```python
from build123d import *

# Parameters (mm, degrees)
ESQUISSE1_R             = 30
BOSS_EXTRU_1_DEPTH      = 15
ESQUISSE2_W             = 9.340839883
ESQUISSE2_H             = 53.061818545
ENL_V_MAT_EXTRU_1_DEPTH = 7
ESQUISSE3_W             = 49.4498788
ESQUISSE3_H             = 120
BOSS_EXTRU_2_DEPTH      = 18
ESQUISSE4_R             = 7
ENL_V_MAT_EXTRU_2_DEPTH = 2
ENL_V_MAT_EXTRU_3_DEPTH = 129.01952976
ESQUISSE6_R             = 10
BOSS_EXTRU_3_DEPTH      = 10
ESQUISSE7_W             = 5
ESQUISSE7_H             = 120
ENL_V_MAT_EXTRU_4_DEPTH = 4
D_POUILLE1_ANGLE        = 40


with BuildPart() as part:
    # Esquisse1 → Boss.-Extru.1 (new body)
    with BuildSketch(Plane.XY):
        Circle(ESQUISSE1_R)
    extrude(amount=BOSS_EXTRU_1_DEPTH)

    # Esquisse2 → Enlèv. mat.-Extru.1 (cut)
    with BuildSketch(Plane.XY.offset(15)):
        with Locations((26.230396322, -0.346809271)):
            Rectangle(ESQUISSE2_W, ESQUISSE2_H)
        with Locations((-26.230396322, -0.346809271)):
            Rectangle(ESQUISSE2_W, ESQUISSE2_H)
    extrude(amount=-ENL_V_MAT_EXTRU_1_DEPTH, mode=Mode.SUBTRACT)

    # Esquisse3 → Boss.-Extru.2 (add)
    with BuildSketch(Plane.XY.offset(15)):
        Rectangle(ESQUISSE3_W, ESQUISSE3_H)
    extrude(amount=BOSS_EXTRU_2_DEPTH)

    # Esquisse4 → Enlèv. mat.-Extru.2 (cut)
    with BuildSketch(Plane.XZ.offset(60)):
        with Locations(Location((12.7249394, 24, 0), (0, 0, 270))):
            Circle(ESQUISSE4_R)
        with Locations(Location((-12.7249394, 24, 0), (0, 0, 270))):
            Circle(ESQUISSE4_R)
    enl_v_mat_extru_2 = extrude(amount=-ENL_V_MAT_EXTRU_2_DEPTH, mode=Mode.SUBTRACT)

    # Symétrie1: Enlèv. mat.-Extru.2 across plane
    add(enl_v_mat_extru_2.mirror(Plane.ZX), mode=Mode.SUBTRACT)

    # Esquisse5 → Enlèv. mat.-Extru.3 (cut, through all)
    with BuildSketch(Plane.XZ.offset(60)):
        with BuildLine():
            Line((24.7249394, 18.33578408), (21.356248325, 18.33578408))
            Line((21.356248325, 18.33578408), (21.356248325, 16.410354936))
            Line((21.356248325, 16.410354936), (21.889577151, 16.410354936))
            ThreePointArc((21.889577151, 16.410354936), (22.243130541, 16.263908326), (22.389577151, 15.910354936))
            Line((22.389577151, 15.910354936), (22.389577151, 15))
            Line((22.389577151, 15), (22.700668624, 13.139727122))
            Line((22.700668624, 13.139727122), (26.027148326, 13.139727122))
            Line((26.027148326, 13.139727122), (26.027148326, 18.33578408))
            Line((26.027148326, 18.33578408), (24.7249394, 18.33578408))
        make_face()
        with BuildLine():
            Line((-22.389577151, 15.910354936), (-22.389577151, 15))
            Line((-22.389577151, 15), (-22.389577151, 13.757493185))
            Line((-22.389577151, 13.757493185), (-25.545793937, 13.757493185))
            Line((-25.545793937, 13.757493185), (-25.842888818, 18.33578408))
            Line((-25.842888818, 18.33578408), (-24.7249394, 18.33578408))
            Line((-24.7249394, 18.33578408), (-21.356248325, 18.33578408))
            Line((-21.356248325, 18.33578408), (-21.356248325, 16.410354936))
            Line((-21.356248325, 16.410354936), (-21.889577151, 16.410354936))
            ThreePointArc((-21.889577151, 16.410354936), (-22.243130541, 16.263908326), (-22.389577151, 15.910354936))
        make_face()
    extrude(amount=-ENL_V_MAT_EXTRU_3_DEPTH, mode=Mode.SUBTRACT)

    # Esquisse6 → Boss.-Extru.3 (add)
    with BuildSketch(Plane(origin=(0, 0, 0), x_dir=(-1, 0, 0), z_dir=(0, 0, -1))):
        with Locations(Location((0, 0, 0), (0, 0, 180))):
            Circle(ESQUISSE6_R)
    extrude(amount=BOSS_EXTRU_3_DEPTH)

    # Esquisse7 → Enlèv. mat.-Extru.4 (cut)
    with BuildSketch(Plane.XY.offset(33)):
        Rectangle(ESQUISSE7_W, ESQUISSE7_H)
    extrude(amount=-ENL_V_MAT_EXTRU_4_DEPTH, mode=Mode.SUBTRACT)

    # Dépouille1
    d_pouille1_faces = [part.faces().sort_by_distance(p)[0] for p in [
        (-2.5, 0, 31),
        (2.5, 0, 31),
    ]]
    draft(d_pouille1_faces, Plane(origin=(-2.5, 60, 29), x_dir=(1, 0, 0), z_dir=(0, 0, 1)), D_POUILLE1_ANGLE)


solid = part.part
```
Model file for the job. Use its own axes, mm. A direction names the side the tool comes from. Coordinates: 2 decimals unless noted, no trailing zeros. Loops run counter-clockwise (first coordinate to the right, second up) from the corner with the lowest first, then second, coordinate; pieces in that order, holes last. Notation, with made-up numbers: (82, 25.5) - (117, 25.5) arc R28 ccw to (117, 62.5) - close; hole circle Ø4 at (71.5, 77). An arc over 180 degrees is marked (long way). Write item = value, one per line. Start each with the question number.
Item 1: Drop flat-ended pins along their axis: pin 1 Ø4 at (x, z) = (13, 11.5) entering from +Y; pin 2 Ø6 at (x, y) = (-16.5, -47) entering from -Z; pin 3 Ø1.5 at (x, y) = (-1, 7) entering from +Z. Give the stop position or say it passes through.
Item 2: Saw through at C-C, the plane y = -46.5. List the corners of the cut face in (x, z), then the cut area to 3 significant figures.
Item 3: Saw through at D-D, the plane y = -18. List the corners of the cut face in (x, z).
Item 4: Pull direction Z, two halves, no side cores. Call faces 1 (the face through (13, -58, 24)), 2 (the face through (-4.202, -0.84, 31.028)), 3 (the face through (0, 0, -10)): +Z half, -Z half, draft (parallel to the pull), parting line (faces both ways), or undercut.
Item 5: 3-axis set-ups, long thin cutter, end or side, ignore diameter. For faces 4 (the face through (8.466, -59.014, 29.555)), 5 (the face through (-25, 0, 8)), 6 (the face through (13, 58, 24)), 7 (the face through (13, 0, 0)), 8 (the face through (21.56, 0, 12)): which of +Z, -Z, +X, -X, +Y, -Y reach the whole face in a straight line?
Item 6: Saw through at A-A, the plane z = 24. List the corners of the cut face in (x, y), then the cut area to 3 significant figures.
Item 7: Saw through at B-B, the plane x = 0. List the corners of the cut face in (y, z), then the cut area to 3 significant figures.
Item 8: Wall check: probe 1 along X at (y, z) = (58.9, 24); probe 2 along Z at (x, y) = (22, -27); probe 3 along Z at (x, y) = (-23.5, -1). Give the ranges that are in metal, low to high. Write a range as [from, to].
Answers:
q1.pin_1 = 27.91
q1.pin_2 = 15
q1.pin_3 = 29
q2.outline = (-24.72, 18.34) - (-21.36, 18.34) - (-21.36, 16.41) - (-21.89, 16.41) arc R0.5 ccw to (-22.39, 15.91) - (-22.39, 15) - (22.39, 15) - (22.39, 15.91) arc R0.5 ccw to (21.89, 16.41) - (21.36, 16.41) - (21.36, 18.34) - (24.72, 18.34) - (24.72, 33) - (5.86, 33) - (2.5, 29) - (-2.5, 29) - (-5.86, 33) - (-24.72, 33) - close
q2.area = 837 mm2
q3.outline = (-24.72, 18.34) - (-21.36, 18.34) - (-21.36, 16.41) - (-21.89, 16.41) arc R0.5 ccw to (-22.39, 15.91) - (-22.39, 15) - (-21.56, 15) - (-21.56, 8) - (-24, 8) - (-24, 0) - (24, 0) - (24, 8) - (21.56, 8) - (21.56, 15) - (22.39, 15) - (22.39, 15.91) arc R0.5 ccw to (21.89, 16.41) - (21.36, 16.41) - (21.36, 18.34) - (24.72, 18.34) - (24.72, 33) - (5.86, 33) - (2.5, 29) - (-2.5, 29) - (-5.86, 33) - (-24.72, 33) - close
q4.face_1 = undercut
q4.face_2 = +Z half
q4.face_3 = -Z half
q5.face_4 = -Y
q5.face_5 = -X, +Y, -Y
q5.face_6 = +Y
q5.face_7 = -Z
q5.face_8 = +X, +Y, -Y
q6.outline = (-24.72, -60) - (-19.72, -60) - (-19.72, -58) - (-5.72, -58) - (-5.72, -60) - (5.72, -60) - (5.72, -58) - (19.72, -58) - (19.72, -60) - (24.72, -60) - (24.72, 60) - (19.72, 60) - (19.72, 58) - (5.72, 58) - (5.72, 60) - (-5.72, 60) - (-5.72, 58) - (-19.72, 58) - (-19.72, 60) - (-24.72, 60) - close
q6.area = 5,820 mm2
q7.outline = (-60, 15) - (-30, 15) - (-30, 0) - (-10, 0) - (-10, -10) - (10, -10) - (10, 0) - (30, 0) - (30, 15) - (60, 15) - (60, 29) - (-60, 29) - close
q7.area = 2,780 mm2
q8.probe_1 = [-24.72, -19.72], [-5.72, 5.72], [19.72, 24.72]
q8.probe_2 = [15, 16.4], [18.34, 33]
q8.probe_3 = [0, 8], [18.34, 33]
